Input: dimensioned drawing with shaded views. Units: mm. Origin: part minimum x, y, z. A direction names the side the tool comes from. Round coordinates to 2 decimals unless told otherwise and drop trailing zeros. Write each loop counter-clockwise with the first axis right and the second up, starting at its lowest first coordinate (ties: lowest second). Pieces come first, ordered by that corner, then holes. Notation, with made-up numbers: M -36.75,9 L 17.25,9 A23 ccw 17.25,43 Z; hole C 88.25,-23 d6. An arc over 180 degrees is marked long. Answer in a Markdown table with one row per item. Add a question column.
Item 1: Set-up query: the marked faces 1, 2, 3 and 4. Return all of +Z, -Z, +X, -X, +Y, -Y with unobstructed straight access to the full face (end or side cutting, diameter ignored); none if empty.
Item 2: Cut plane B-B on x = 3.75. Return loops of the section in (y, z).
Item 3: Material intervals for probe 1 along Y at (x, z) = (11.5, 3.2); probe 2 along Z at (x, y) = (8.5, 10), sorted ascending.
Item 4: Contact query for flat-ended pins moving along their axis: pin 1 (0.8 mm diameter, centred on x = 8.5, z = 5.5, fed in from +Y); pin 2 (2 mm diameter, centred on y = 5, z = 4.5, fed in from +X); pin 3 (2 mm diameter, centred on y = 5.5, z = 3.5, fed in from -X). Output: stop coordinate, or through.
Item 5: Cut plane C-C on z = 3.5. Return loops of the section in (x, y), and give its area (3 significant figures).
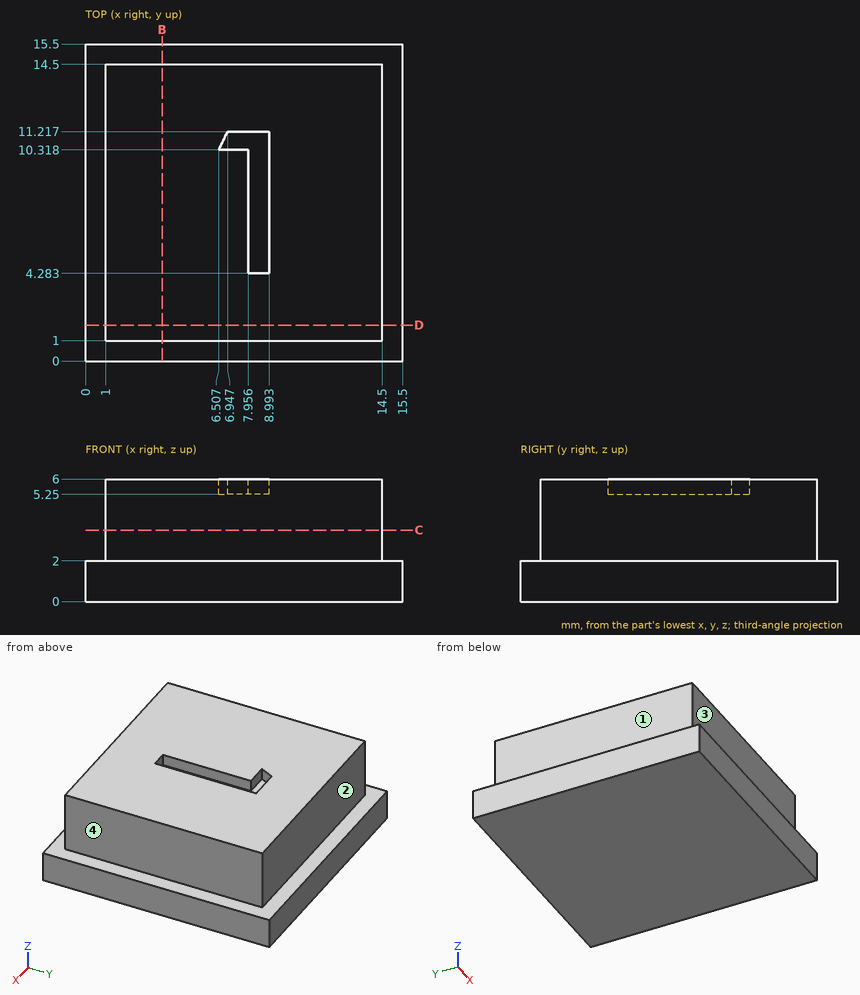
Results below:
| question | item | result |
|---|---|---|
| 1 | face 1 | +Z, -X, +Y, -Y |
| 1 | face 2 | +Z, +X, -X, +Y |
| 1 | face 3 | +Z, +X, -X, -Y |
| 1 | face 4 | +Z, +X, +Y, -Y |
| 2 | outline | M 0,0 L 15.5,0 L 15.5,2 L 14.5,2 L 14.5,6 L 1,6 L 1,2 L 0,2 Z |
| 3 | probe 1 | 1 to 14.5 |
| 3 | probe 2 | 0 to 5.25 |
| 4 | pin 1 | y = 14.5 |
| 4 | pin 2 | x = 14.5 |
| 4 | pin 3 | x = 1 |
| 5 | outline | M 1,1 L 14.5,1 L 14.5,14.5 L 1,14.5 Z |
| 5 | area | 182 mm2 |
